Here's how the part is built. I have some questions about the finished solid (model axes, mm). A direction names the side the tool comes from. Round coordinates to 2 decimals unless told otherwise and drop trailing zeros. Loops run counter-clockwise (first coordinate to the right, second up) from the corner with the lowest first, then second, coordinate; pieces in that order, holes last. Notation, with made-up numbers: M -17.5,-3.75 L 39.5,-3.75 A17 ccw 39.5,0.25 Z; hole C 8,84.25 d4. An arc over 180 degrees is marked long. Answer as CSV lines item,"result".
```python
from build123d import *

# Parameters (mm, degrees)
SKIZZE1_W                       = 21
SKIZZE1_H                       = 20
SKIZZE1_R                       = 5
SKIZZE1_R_2                     = 1.25
AUFSATZ_LINEAR_AUSTRAGEN1_DEPTH = 2.5
SCHNITT_LINEAR_START            = 2.5
SCHNITT_LINEAR_AUSTRAGEN1_DEPTH = 2.5
SKIZZE4_R                       = 0.75
SCHNITT_LINEAR_AUSTRAGEN2_DEPTH = 3


with BuildPart() as part:
    # Skizze1 → Aufsatz-Linear austragen1 (new body, symmetric)
    with BuildSketch(Plane.XY):
        Rectangle(SKIZZE1_W, SKIZZE1_H)
        Circle(SKIZZE1_R, mode=Mode.SUBTRACT)
        with Locations((6.92820323, 4)):
            Circle(SKIZZE1_R_2, mode=Mode.SUBTRACT)
        with Locations((-6.92820323, -4)):
            Circle(SKIZZE1_R_2, mode=Mode.SUBTRACT)
        with Locations((-6.92820323, 4)):
            Circle(SKIZZE1_R_2, mode=Mode.SUBTRACT)
        with Locations((6.92820323, -4)):
            Circle(SKIZZE1_R_2, mode=Mode.SUBTRACT)
    extrude(amount=AUFSATZ_LINEAR_AUSTRAGEN1_DEPTH, both=True)

    # Skizze1<3> → Schnitt-Linear austragen1 (cut)
    with BuildSketch(Plane.XY.offset(SCHNITT_LINEAR_START)):
        with BuildLine():
            Line((-6.92820323, 6.5), (6.92820323, 6.5))
            ThreePointArc((6.92820323, 6.5), (8.695970183, 5.767766953), (9.42820323, 4))
            Line((9.42820323, 4), (9.42820323, -4))
            ThreePointArc((9.42820323, -4), (8.695970183, -5.767766953), (6.92820323, -6.5))
            Line((6.92820323, -6.5), (-6.92820323, -6.5))
            ThreePointArc((-6.92820323, -6.5), (-8.695970183, -5.767766953), (-9.42820323, -4))
            Line((-9.42820323, -4), (-9.42820323, 4))
            ThreePointArc((-9.42820323, 4), (-8.695970183, 5.767766953), (-6.92820323, 6.5))
        make_face()
    extrude(amount=-SCHNITT_LINEAR_AUSTRAGEN1_DEPTH, mode=Mode.SUBTRACT)

    # Skizze4 → Schnitt-Linear austragen2 (cut)
    with BuildSketch(Plane(origin=(0, 10, 0), x_dir=(1, 0, 0), z_dir=(0, 1, 0))):
        with Locations((-4.25, 0)):
            Circle(SKIZZE4_R)
        with Locations((4.25, 0)):
            Circle(SKIZZE4_R)
    schnitt_linear_austragen2 = extrude(amount=-SCHNITT_LINEAR_AUSTRAGEN2_DEPTH, mode=Mode.SUBTRACT)

    # Spiegeln1: Schnitt-Linear austragen2 across plane
    add(schnitt_linear_austragen2.mirror(Plane.ZX), mode=Mode.SUBTRACT)


solid = part.part
```
1. We'd pull the mould along X, two halves only. Please class faces 6 (the flat face through (10.5, 0, 0)), 7 (the cylindrical face through (-5, -9, 0)), 8 (the flat face through (0, 10, 0)), 9 (the cylindrical face through (-6.35, 2.89, -1.27)): pulls with the +X half, pulls with the -X half, needs draft (parallel to the pull), parting line crosses it, or undercut.
Evaluation:
face 6,"pulls with the +X half"
face 7,"undercut"
face 8,"needs draft"
face 9,"undercut"
2. Which directions (+Z, -Z, +X, -X, +Y, -Y) give clear straight access to the entire face, cutting with the end or side of a thin tool? Please do faces 1 (the flat face through (4, -7, 0)), 2 (the cylindrical face through (-8.676, -5.787, 1.268)), 3 (the cylindrical face through (5.936, -4.761, -1.268)), 4 (the flat face through (-2, 5, -2.5)), 5 (the cylindrical face through (3.655, 8.521, 0.456)).
Evaluation:
face 1,"-Y"
face 2,"+Z"
face 3,"+Z, -Z"
face 4,"-Z, +X, -X, +Y, -Y"
face 5,"+Y"
3. I want a section at D-D, the plane x = -0.75. Please give me the cut outline in (y, z).
Evaluation:
outline,"M -10,-2.5 L -4.94,-2.5 L -4.94,0 L -6.5,0 L -6.5,2.5 L -10,2.5 Z; M 4.94,-2.5 L 10,-2.5 L 10,2.5 L 6.5,2.5 L 6.5,0 L 4.94,0 Z"
4. I want a section at A-A, the plane y = 0. Please give me the cut outline in (x, z), and give its area (3 significant figures).
Evaluation:
outline,"M -10.5,-2.5 L -5,-2.5 L -5,0 L -9.43,0 L -9.43,2.5 L -10.5,2.5 Z; M 5,-2.5 L 10.5,-2.5 L 10.5,2.5 L 9.43,2.5 L 9.43,0 L 5,0 Z"
area,"32.9 mm²"
5. I want a section at C-C, the plane z = 1.3. Please give me the cut outline in (x, y).
Evaluation:
outline,"M -10.5,-10 L 10.5,-10 L 10.5,10 L -10.5,10 Z; hole M -9.43,-4 A2.5 ccw -6.93,-6.5 L 6.93,-6.5 A2.5 ccw 9.43,-4 L 9.43,4 A2.5 ccw 6.93,6.5 L -6.93,6.5 A2.5 ccw -9.43,4 Z"
6. For P1, Ø1.2, axis at x = 4.5, z = 0, coming from the +Y side; P2, Ø1.2, axis at x = 4.25, z = 0, coming from the +Y side; P3, Ø10, axis at x = -2.5, y = 1, coming from the +Z side; P4, Ø2, axis at x = 6.93, y = -4, coming from the +Z side, each with a flat end and sliding along its axis, tell me the tip position at first contact or that it passes through.
Evaluation:
P1,"stops at y = 10"
P2,"stops at y = 7"
P3,"stops at z = 0"
P4,"passes through"
7. If I drill on line 1 (X direction, y = -8.6, z = 0); line 2 (Y direction, x = -4.5, z = 1.6); line 3 (Z direction, x = 4.25, y = 8.65), over which ranges is the centre line in solid material (lowest first)? Write a range as [from, to].
Evaluation:
line 1,"x = [-10.5, -5], [-3.5, 3.5], [5, 10.5]"
line 2,"y = [-10, -6.5], [6.5, 10]"
line 3,"z = [-2.5, -0.75], [0.75, 2.5]"
8. I want a section at B-B, the plane z = -1. Please give me the cut outline in (x, y).
Evaluation:
outline,"M -10.5,-10 L 10.5,-10 L 10.5,10 L -10.5,10 Z; hole C -6.93,-4 d2.5; hole C -6.93,4 d2.5; hole C 0,0 d10; hole C 6.93,-4 d2.5; hole C 6.93,4 d2.5"
